from build123d import *

# Parameters (mm, degrees)
BOSS_EXTRUDE1_DEPTH                            = 8
SKETCH8_W                                      = 50
SKETCH8_H                                      = 68
SKETCH8_W_2                                    = 10
SKETCH8_H_2                                    = 75
CUT_EXTRUDE2_DEPTH                             = 9
F_9_16_12_TAPPED_HOLE1_D                       = 12.30376
FILLET1_R                                      = 3
M4_CLEARANCE_HOLE1_D                           = 4.5
SKETCH7_R                                      = 9.0297
CUT_EXTRUDE1_DEPTH                             = 1.27
F_4_40_TAPPED_HOLE1_D                          = 2.2606
CUT_EXTRUDE3_DEPTH                             = 1.27
FILLET2_R                                      = 3.175
FILLET2_OF_MIRROR1_R                           = 3.175
CBORE_FOR_4_SOCKET_HEAD_CAP_SCREW1_D           = 3.2639
CBORE_FOR_4_SOCKET_HEAD_CAP_SCREW1_CBORE_D     = 5.55752
CBORE_FOR_4_SOCKET_HEAD_CAP_SCREW1_CBORE_DEPTH = 5.999999938
F_6_32_TAPPED_HOLE2_D                          = 2.7051
F_6_32_TAPPED_HOLE2_DEPTH                      = 10.97
F_6_32_TAPPED_HOLE2_TIP                        = 0.81269403


with BuildPart() as part:
    # Sketch1 → Boss-Extrude1 (new body)
    with BuildSketch(Plane(origin=(0, 0, 0), x_dir=(1, 0, 0), z_dir=(0, 1, 0))):
        with BuildLine():
            Line((62.5, -85), (62.5, 62.5))
            Line((62.5, 62.5), (17.267202684, 62.5))
            Line((17.267202684, 62.5), (9.08736201, 89.173709584))
            ThreePointArc((9.08736201, 89.173709584), (0, 95), (-9.08736201, 89.173709584))
            Line((-9.08736201, 89.173709584), (-17.267202684, 62.5))
            Line((-17.267202684, 62.5), (-62.5, 62.5))
            Line((-62.5, 62.5), (-62.5, -85))
            ThreePointArc((-62.5, -85), (-52.5, -95), (-42.5, -85))
            Line((-42.5, -85), (-42.5, -62.5))
            Line((-42.5, -62.5), (42.5, -62.5))
            Line((42.5, -62.5), (42.5, -85))
            ThreePointArc((42.5, -85), (52.5, -95), (62.5, -85))
        make_face()
    extrude(amount=-BOSS_EXTRUDE1_DEPTH)

    # Sketch8 → Cut-Extrude2 (cut, through all)
    with BuildSketch(Plane(origin=(0, 0, 0), x_dir=(1, 0, 0), z_dir=(0, 1, 0))):
        Rectangle(SKETCH8_W, SKETCH8_H)
        with Locations((-57.5, 0)):
            Rectangle(SKETCH8_W_2, SKETCH8_H_2)
        with Locations((57.5, 0)):
            Rectangle(SKETCH8_W_2, SKETCH8_H_2)
    extrude(amount=-CUT_EXTRUDE2_DEPTH, mode=Mode.SUBTRACT)

    # 9/16-12 Tapped Hole1 (through all)
    with Locations(Plane(origin=(-52.5, 0, 85), x_dir=(0, 0, 1), z_dir=(0, 1, 0))):
        with Locations((0, 0), (-170, 52.5), (0, 105)):
            Hole(F_9_16_12_TAPPED_HOLE1_D / 2)

    # Fillet1
    fillet1_edges = [part.edges().sort_by_distance(p)[0] for p in [
        (17.267202684, -4, -62.5),
        (62.5, -4, -62.5),
        (42.5, -4, 62.5),
        (-42.5, -4, 62.5),
        (-62.5, -4, -62.5),
        (-17.267202684, -4, -62.5),
        (-25, -4, 34),
        (-25, -4, -34),
        (25, -4, -34),
        (25, -4, 34),
        (-62.5, -4, 37.5),
        (-62.5, -4, -37.5),
        (-52.5, -4, -37.5),
        (-52.5, -4, 37.5),
        (62.5, -4, -37.5),
        (62.5, -4, 37.5),
        (52.5, -4, 37.5),
        (52.5, -4, -37.5),
    ]]
    fillet(fillet1_edges, radius=FILLET1_R)

    # M4 Clearance Hole1 (through all)
    with Locations(Plane(origin=(0, 0, 0), x_dir=(1, 0, 0), z_dir=(0, 1, 0))):
        with Locations((-35.745, 0), (35.745, -35.829), (35.745, 35.829)):
            Hole(M4_CLEARANCE_HOLE1_D / 2)

    # Sketch7 → Cut-Extrude1 (cut)
    with BuildSketch(Plane(origin=(0, 0, 0), x_dir=(1, 0, 0), z_dir=(0, 1, 0))):
        with Locations(Location((-35.745, 0, 0), (0, 0, 270))):  # turned: the seam where the file's is
            Circle(SKETCH7_R)
        with Locations(Location((35.745, 35.829, 0), (0, 0, 270))):  # turned: the seam where the file's is
            Circle(SKETCH7_R)
        with Locations(Location((35.745, -35.829, 0), (0, 0, 270))):  # turned: the seam where the file's is
            Circle(SKETCH7_R)
    extrude(amount=-CUT_EXTRUDE1_DEPTH, mode=Mode.SUBTRACT)

    # #4-40 Tapped Hole1 (through all)
    with Locations(Plane(origin=(0, 0, 0), x_dir=(1, 0, 0), z_dir=(0, 1, 0))):
        with Locations((-59.5, 59.5), (59.5, 59.5), (59.5, -59.5), (-59.5, -59.5)):
            Hole(F_4_40_TAPPED_HOLE1_D / 2)

    # Sketch11 → Cut-Extrude3 (cut)
    with BuildSketch(Plane(origin=(0, 0, 0), x_dir=(1, 0, 0), z_dir=(0, 1, 0))):
        with BuildLine():
            Line((-62.5, 47.5), (-47.5, 62.5))
            Line((-47.5, 62.5), (-59.5, 62.5))
            ThreePointArc((-59.5, 62.5), (-61.621320344, 61.621320344), (-62.5, 59.5))
            Line((-62.5, 59.5), (-62.5, 47.5))
        make_face()
        Polygon((-62.5, -47.5), (-44.5, -65.5), (-62.5, -65.5), align=None)
    cut_extrude3 = extrude(amount=-CUT_EXTRUDE3_DEPTH, mode=Mode.SUBTRACT)

    # Fillet2
    fillet2_edges = [part.edges().sort_by_distance(p)[0] for p in [
        (-44.5, -0.635, 65.5),
    ]]
    fillet(fillet2_edges, radius=FILLET2_R)

    # Mirror1: Cut-Extrude3 across plane
    add(cut_extrude3.mirror(Plane(origin=(0, 0, 0), x_dir=(0, 0, 1), z_dir=(1, 0, 0))), mode=Mode.SUBTRACT)

    # Fillet2 of Mirror1
    fillet2_of_mirror1_edges = [part.edges().sort_by_distance(p)[0] for p in [
        (44.5, -0.635, 65.5),
    ]]
    fillet(fillet2_of_mirror1_edges, radius=FILLET2_OF_MIRROR1_R)

    # Sketch13 → #6-32 Tapped Hole1 (revolve, cut)
    with BuildSketch(Plane(origin=(62.5, -4.825, -50.025), x_dir=(0, 0, -1), z_dir=(0, 1, 0))):
        Polygon((0, 0), (0, 11.78269403), (1.35255, 10.97), (1.35255, 0), align=None)
    f_6_32_tapped_hole1 = revolve(axis=Axis((68.85, -4.825, -50.025), (-1, 0, 0)), mode=Mode.SUBTRACT)

    # Mirror2: #6-32 Tapped Hole1 across plane
    add(f_6_32_tapped_hole1.mirror(Plane(origin=(0, 0, 0), x_dir=(0, 0, 1), z_dir=(1, 0, 0))), mode=Mode.SUBTRACT)

    # CBORE for #4 Socket Head Cap Screw1 (through all)
    with Locations(Plane(origin=(0, 0, 0), x_dir=(1, 0, 0), z_dir=(0, 1, 0))):
        with Locations((-28.276, 43.752), (27.724, 43.752), (27.724, -40.248), (-28.276, -40.248)):
            CounterBoreHole(CBORE_FOR_4_SOCKET_HEAD_CAP_SCREW1_D / 2, CBORE_FOR_4_SOCKET_HEAD_CAP_SCREW1_CBORE_D / 2, CBORE_FOR_4_SOCKET_HEAD_CAP_SCREW1_CBORE_DEPTH)

    # #6-32 Tapped Hole2
    with Locations(Plane.XY.offset(62.5)):
        with Locations((0, -4.825)):
            Hole(F_6_32_TAPPED_HOLE2_D / 2, depth=F_6_32_TAPPED_HOLE2_DEPTH)
            with Locations((0, 0, -(F_6_32_TAPPED_HOLE2_DEPTH + F_6_32_TAPPED_HOLE2_TIP / 2))):  # 118° drill point
                Cone(0, F_6_32_TAPPED_HOLE2_D / 2, F_6_32_TAPPED_HOLE2_TIP, mode=Mode.SUBTRACT)


solid = part.part
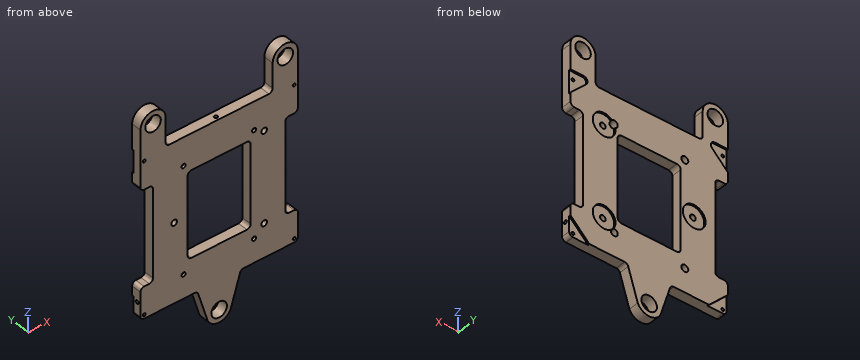
CAD build for the part. Positions are in the model's coordinates, mm. Give positions to 0.01 mm unless a question says otherwise; leave off trailing zeros. Order: outer loops, then holes, each group sorted by start corner. A loop starts at its lowest first (then second) coordinate and runs counter-clockwise, first axis right, second up. Notation, with made-up numbers: (-30, -19.75) - (6, -19.75) arc R21 ccw to (6, -4.75) - close; hole circle Ø1 at (16.5, 19.5). An arc over 180 degrees is marked (long way). Write each question's results on one line, items separated by ' | '.
1. Pin check, flat tips, straight feed: pin 1 (7 mm diameter, centred on x = 35.745, z = -35.829, fed in from +Y); pin 2 (2 mm diameter, centred on y = -4.825, z = -50.025, fed in from -X); pin 3 (6 mm diameter, centred on x = -34, z = -67.5, fed in from +Y); pin 4 (1 mm diameter, centred on x = 43, z = 62, fed in from +Y). Stop position of each tip, or through.
Calculated:
pin 1: stops at y = -1.27 | pin 2: stops at x = -51.32 | pin 3: passes through | pin 4: stops at y = 0
2. Probe L1, parallel to X at y = -3.75, z = 85; L2, parallel to X at y = -1.5, z = -7; L3, parallel to Z at x = -28.5, y = -0.25. List the from-to ranges inside material, lowest first. Write a range as from..to.
Calculated:
L1: x = -62.5..-58.65, -46.35..-42.5, 42.5..46.35, 58.65..62.5 | L2: x = -52.5..-25, 25..52.5 | L3: z = -62.5..-46.52, -40.98..-5.39, 5.39..37.48, 43.02..62.5
3. Saw through at B-B on z = -72. List the corners of the cut face in (x, y), and give its area (3 significant figures).
Calculated:
outline: (-14.35, -8) - (14.35, -8) - (14.35, 0) - (-14.35, 0) - close | area: 230 mm2
4. Saw through at A-A on z = 54.5. List the corners of the cut face in (x, y) (3 decimals).
Calculated:
outline: (-62.5, -8) - (62.5, -8) - (62.5, -1.27) - (55.5, -1.27) - (55.5, 0) - (-55.5, 0) - (-55.5, -1.27) - (-62.5, -1.27) - close; hole circle Ø2.705 at (0, -4.825)
